Could you check a few things on this model? Use its own coordinates, in mm. Give positions to 0.01 mm unless a question says otherwise; leave off trailing zeros. Loops run counter-clockwise (first coordinate to the right, second up) from the corner with the lowest first, then second, coordinate; pieces in that order, holes last. Notation, with made-up numbers: (-30, 26) - (20, 26) arc R18 ccw to (20, 42) - close; hole circle Ø11 at (62, 75.5). An arc over 180 degrees is marked (long way). Use CSV: the item, a comma, the result in double quotes.
from build123d import *

# Parameters (mm, degrees)
SKETCH1_R           = 11.1125
BOSS_EXTRUDE1_DEPTH = 6.35
FILLET1_R           = 12.7


with BuildPart() as part:
    # Sketch1 → Boss-Extrude1 (new body)
    with BuildSketch(Plane.XY):
        Polygon((20.207363698, 1349.509753019), (-183.500636302, 1349.509753019), (-183.500636302, 1528.897253019), (-284.846636302, 1528.897253019), (-284.846636302, 1732.605253019), (-183.500636302, 1732.605253019), (-183.500636302, 1911.992753019), (20.207363698, 1911.992753019), (20.207363698, 1732.605253019), (121.553363698, 1732.605253019), (121.553363698, 1528.897253019), (20.207363698, 1528.897253019), align=None)
        with Locations((-139.050636302, 1867.542753019)):
            Circle(SKETCH1_R, mode=Mode.SUBTRACT)
        with Locations((-151.496636302, 1694.505253019)):
            Circle(SKETCH1_R, mode=Mode.SUBTRACT)
        with Locations(Location((-11.796636302, 1694.505253019, 0), (0, 0, 180))):
            Circle(SKETCH1_R, mode=Mode.SUBTRACT)
        with Locations(Location((-24.242636302, 1867.542753019, 0), (0, 0, 180))):
            Circle(SKETCH1_R, mode=Mode.SUBTRACT)
        with Locations((-24.242636302, 1393.959753019)):
            Circle(SKETCH1_R, mode=Mode.SUBTRACT)
        with Locations(Location((-139.050636302, 1393.959753019, 0), (0, 0, 180))):
            Circle(SKETCH1_R, mode=Mode.SUBTRACT)
        with Locations(Location((-151.496636302, 1566.997253019, 0), (0, 0, 180))):
            Circle(SKETCH1_R, mode=Mode.SUBTRACT)
        with Locations((-11.796636302, 1566.997253019)):
            Circle(SKETCH1_R, mode=Mode.SUBTRACT)
        with Locations((-240.396636302, 1694.505253019)):
            Circle(SKETCH1_R, mode=Mode.SUBTRACT)
        with Locations((-139.050636302, 1778.642753019)):
            Circle(SKETCH1_R, mode=Mode.SUBTRACT)
        with Locations(Location((-139.050636302, 1482.859753019, 0), (0, 0, 180))):
            Circle(SKETCH1_R, mode=Mode.SUBTRACT)
        with Locations(Location((-240.396636302, 1566.997253019, 0), (0, 0, 180))):
            Circle(SKETCH1_R, mode=Mode.SUBTRACT)
        with Locations(Location((-24.242636302, 1778.642753019, 0), (0, 0, 180))):
            Circle(SKETCH1_R, mode=Mode.SUBTRACT)
        with Locations(Location((77.103363698, 1694.505253019, 0), (0, 0, 180))):
            Circle(SKETCH1_R, mode=Mode.SUBTRACT)
        with Locations((77.103363698, 1566.997253019)):
            Circle(SKETCH1_R, mode=Mode.SUBTRACT)
        with Locations((-24.242636302, 1482.859753019)):
            Circle(SKETCH1_R, mode=Mode.SUBTRACT)
    extrude(amount=BOSS_EXTRUDE1_DEPTH)

    # Fillet1
    fillet1_edges = [part.edges().sort_by_distance(p)[0] for p in [
        (-183.500636302, 1528.897253019, 3.175),
        (-183.500636302, 1732.605253019, 3.175),
        (20.207363698, 1732.605253019, 3.175),
        (20.207363698, 1528.897253019, 3.175),
    ]]
    fillet(fillet1_edges, radius=FILLET1_R)


solid = part.part
1) Suppose I cut it at C-C (x = -221). Please give me the cut outline in (y, z).
Answer below:
outline,"(1528.9, 0) - (1732.61, 0) - (1732.61, 6.35) - (1528.9, 6.35) - close"
2) Suppose I cut it at A-A (z = 2.5). State how many separate pieces and enclosed holes the cut face has, plus the area to 3 significant figures.
Answer below:
separate pieces,"1"
enclosed holes,"16"
area,"150,000 mm2"
3) We'd pull the mould along X, two halves only. Please class faces 1 (the cylindrical face through (23.83, 1525.08, 3.22)), 2 (the cylindrical face through (-187.32, 1736.227, 3.219)), 3 (the cylindrical face through (-238.95, 1555.98, 3.13)), 4 (the flat face through (-79, 1635, 0)): +X half, -X half, draft (parallel to the pull), parting line (faces both ways), or undercut.
Answer below:
face 1,"+X half"
face 2,"-X half"
face 3,"undercut"
face 4,"draft"
4) I need wall thicknesses on line 1 along X through (y, z) = (1778.5, 1.25); line 2 along Y through (x, z) = (-248.5, 1); line 3 along Y through (x, z) = (72, 3.25). Which ranges of each line are inside material? Lowest first, please.
Answer below:
line 1,"x = -183.5 to -150.16, -127.94 to -35.35, -13.13 to 20.21"
line 2,"y = 1528.9 to 1559.39, 1574.6 to 1686.9, 1702.11 to 1732.61"
line 3,"y = 1528.9 to 1557.13, 1576.87 to 1684.63, 1704.38 to 1732.61"
5) Suppose I cut it at B-B (y = 1833). Please give me the cut outline in (x, z), plus the area to 3 significant figures.
Answer below:
outline,"(-183.5, 0) - (20.21, 0) - (20.21, 6.35) - (-183.5, 6.35) - close"
area,"1,290 mm2"
6) I'm going to push flat-ended pins straight in: P1, Ø3, axis at x = 64.5, z = 5.5, coming from the -Y side; P2, Ø20, axis at x = -24.24, y = 1867.54, coming from the -Z side; P3, Ø1.9, axis at x = 90.5, z = 4.5, coming from the +Y side. Where does each tip first touch, or does it pass through?
Answer below:
P1,"stops at y = 1528.9"
P2,"passes through"
P3,"stops at y = 1732.61"
